Verification items for the finished model (mm, model axes). A direction names the side the tool comes from. Round coordinates to 2 decimals unless told otherwise and drop trailing zeros. Write each loop counter-clockwise with the first axis right and the second up, starting at its lowest first coordinate (ties: lowest second). Pieces come first, ordered by that corner, then holes. Notation, with made-up numbers: (61, -21) - (68, -21) arc R29 cw to (68, -1) - close; hole circle Ø11 at (54, -16). An arc over 180 degrees is marked (long way). Answer as a JSON object with one key per item and string values.
```python
from build123d import *

# Parameters (mm, degrees)
F0_W     = 10.16
F0_H     = 5.08
F0_W_2   = 3.2
F0_H_2   = 3.2
F1_DEPTH = 5.08
F2_W     = 4.572
F2_H     = 5.08
F3_DEPTH = 3.84


with BuildPart() as f1:
    # F0 (on Front) → F1 (new body)
    with BuildSketch(Plane.XZ):
        with Locations((14.68, 11.46)):
            Rectangle(F0_W, F0_H)
        with BuildLine():
            ThreePointArc((0, 1.27), (0.371974, 0.371974), (1.27, 0))
            Line((1.27, 0), (3.2, 0))
            Line((3.2, 0), (3.2, 3.2))
            Line((3.2, 3.2), (3.2, 10.8))
            Line((3.2, 10.8), (0, 10.8))
            Line((0, 10.8), (0, 1.27))
        make_face()
        with Locations((4.8, 1.6)):
            Rectangle(F0_W_2, F0_H_2)
        with BuildLine():
            Line((6.4, 3.2), (6.4, 0))
            Line((6.4, 0), (8.33, 0))
            ThreePointArc((8.33, 0), (9.228026, 0.371974), (9.6, 1.27))
            Line((9.6, 1.27), (9.6, 8.92))
            Line((9.6, 8.92), (9.6, 14))
            Line((9.6, 14), (6.4, 14))
            Line((6.4, 14), (6.4, 3.2))
        make_face()
        with BuildLine():
            Line((0, 0), (1.27, 0))
            ThreePointArc((1.27, 0), (0.371974, 0.371974), (0, 1.27))
            Line((0, 1.27), (0, 0))
        make_face()
        with BuildLine():
            ThreePointArc((9.6, 1.27), (9.228026, 0.371974), (8.33, 0))
            Line((8.33, 0), (9.6, 0))
            Line((9.6, 0), (9.6, 1.27))
        make_face()
        with BuildLine():
            Line((0, 12.73), (0, 10.8))
            Line((0, 10.8), (3.2, 10.8))
            Line((3.2, 10.8), (3.2, 14))
            Line((3.2, 14), (1.27, 14))
            ThreePointArc((1.27, 14), (0.371974, 13.628026), (0, 12.73))
        make_face()
        with BuildLine():
            Line((0, 14), (0, 12.73))
            ThreePointArc((0, 12.73), (0.371974, 13.628026), (1.27, 14))
            Line((1.27, 14), (0, 14))
        make_face()
    extrude(amount=F1_DEPTH)

    # F2 (on face) → F3 (join)
    with BuildSketch(Plane(origin=(0, 0, 8.92), x_dir=(1, 0, 0), z_dir=(0, 0, -1))):
        with Locations((17.474, 2.54)):
            Rectangle(F2_W, F2_H)
    extrude(amount=F3_DEPTH)


solid = f1.part
```
1. Cross-section at C-C (z = 1). Record the boundary of the cut face in (x, y).
Completed:
{"outline": "(0, -5.08) - (9.6, -5.08) - (9.6, 0) - (0, 0) - close"}
2. Material ranges on probe 1 along X at (y, z) = (-1.9, 6); probe 2 along X at (y, z) = (-3, 10.25); probe 3 along X at (y, z) = (-4.7, 2), recorded low to high. Write a range as from..to.
Completed:
{"probe 1": "x = 0..3.2, 6.4..9.6, 15.19..19.76", "probe 2": "x = 0..3.2, 6.4..19.76", "probe 3": "x = 0..9.6"}
3. Cross-section at D-D (x = 13). Record the boundary of the cut face in (y, z).
Completed:
{"outline": "(-5.08, 8.92) - (0, 8.92) - (0, 14) - (-5.08, 14) - close"}
4. Go/stop test with a flat-tipped pin: pin 1 (1.4 mm diameter, centred on x = 18.5, y = -2.5, fed in from -Z). Record where the tip stops, or that it passes through.
Completed:
{"pin 1": "stops at z = 5.08"}
5. Cross-section at B-B (y = -2.2). Record the boundary of the cut face in (x, z).
Completed:
{"outline": "(0, 0) - (9.6, 0) - (9.6, 8.92) - (15.19, 8.92) - (15.19, 5.08) - (19.76, 5.08) - (19.76, 14) - (6.4, 14) - (6.4, 3.2) - (3.2, 3.2) - (3.2, 14) - (0, 14) - close"}
6. Mould release check, pull along X, two halves, no side actions. Record for faces 1 (the face through (6.4, -3, 9)), 2 (the face through (19.76, -3, 10)), 3 (the face through (8, -5.08, 9)), 4 (the face through (0, -3, 7)): released by +X, released by -X, zero draft, split by the parting line, or undercut.
Completed:
{"face 1": "undercut", "face 2": "released by +X", "face 3": "zero draft", "face 4": "released by -X"}
7. Cross-section at A-A (z = 9.25). Record the boundary of the cut face in (x, y), plus the area to 3 significant figures.
Completed:
{"outline": "(0, -5.08) - (3.2, -5.08) - (3.2, 0) - (0, 0) - close; (6.4, -5.08) - (19.76, -5.08) - (19.76, 0) - (6.4, 0) - close", "area": "84.1 mm^2"}
8. Access from +Z, -Z, +X, -X, +Y, -Y to the whole of each face (thin tool, end or side, straight path). Record for faces 5 (the face through (17, -3, 5.08)), 6 (the face through (15.188, -3, 7)), 7 (the face through (5, -3, 3.2)).
Completed:
{"face 5": "-Z, +X, +Y, -Y", "face 6": "-Z, +Y, -Y", "face 7": "+Z, +Y, -Y"}
